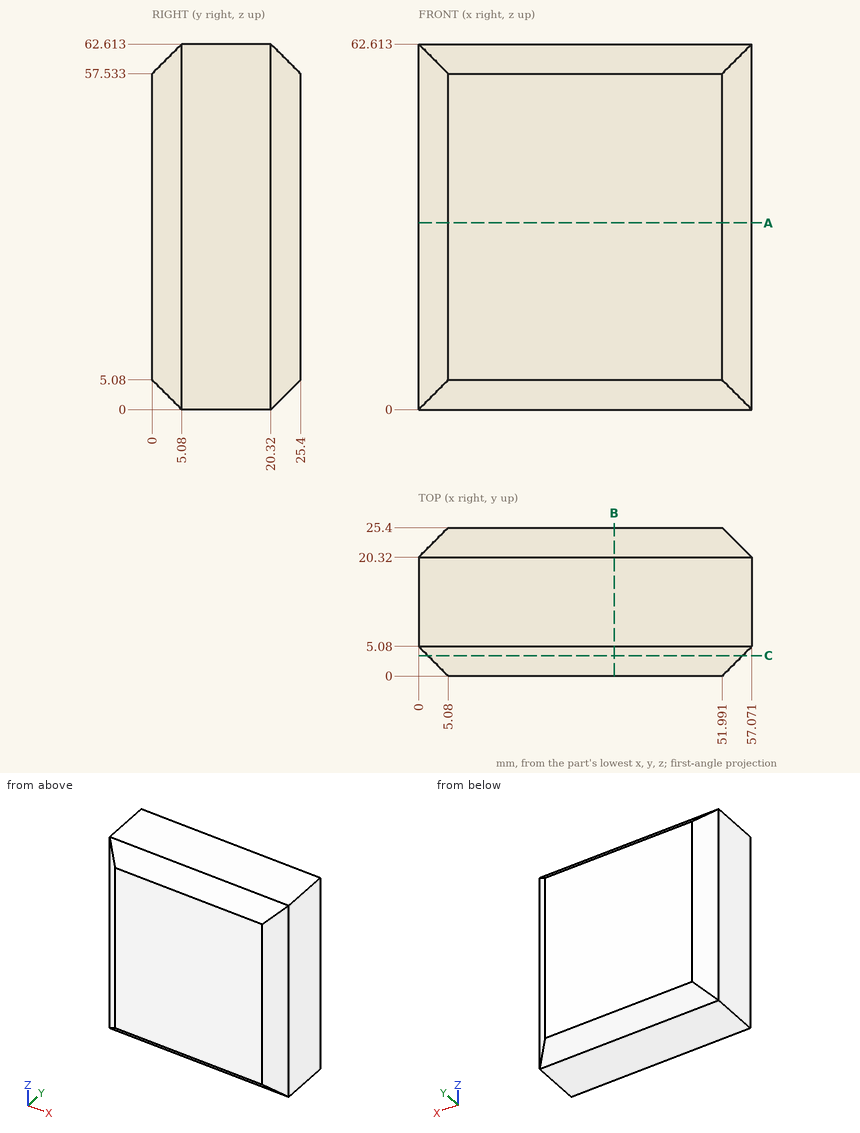
Answer from the drawing. Dimensions are ordinates in mm from the lowest x, y and z of the part. Give positions to 0.01 mm unless a question says otherwise; leave off trailing zeros. Loops run counter-clockwise (first coordinate to the right, second up) from the corner with the lowest first, then second, coordinate; pieces in that order, holes last. Notation, with made-up numbers: (50.5, 30.25) -> (85.5, 30.25) arc R26 ccw to (85.5, 44.25) -> close; hole circle Ø2 at (22.5, 0.5). An arc over 180 degrees is marked (long way). Answer as CSV lines item,"result".
Item 1: Find section C-C on y = 3.5. Give the vertices of the cut face in (x, z).
Returned:
outline,"(1.58, 1.58) -> (55.49, 1.58) -> (55.49, 61.03) -> (1.58, 61.03) -> close"
Item 2: Consider line 1 (Y direction, x = 17, z = 5); line 2 (X direction, y = 1, z = 23.5); line 3 (X direction, y = 1.75, z = 20.5). Determine where each line is inside the solid, lowest interval first. Write a range as [from, to].
Returned:
line 1,"y = [0.08, 25.32]"
line 2,"x = [4.08, 52.99]"
line 3,"x = [3.33, 53.74]"
Item 3: Find section A-A on z = 32. Give the vertices of the cut face in (x, y).
Returned:
outline,"(0, 5.08) -> (5.08, 0) -> (51.99, 0) -> (57.07, 5.08) -> (57.07, 20.32) -> (51.99, 25.4) -> (5.08, 25.4) -> (0, 20.32) -> close"
Item 4: Find section B-B on x = 33.5. Give the vertices of the cut face in (y, z), plus the area to 3 significant figures.
Returned:
outline,"(0, 5.08) -> (5.08, 0) -> (20.32, 0) -> (25.4, 5.08) -> (25.4, 57.53) -> (20.32, 62.61) -> (5.08, 62.61) -> (0, 57.53) -> close"
area,"1,540 mm²"
Item 5: This flat-tipped pin is pushed along its axis until it touches: pin 1 (1.5 mm diameter, centred on x = 51.5, y = 22, fed in from -Z). Where does it stop, or does it pass through?
Returned:
pin 1,"stops at z = 0.93"
